from build123d import *

# Parameters (mm, degrees)
F0_W      = 500
F0_H      = 240
F0_W_2    = 420
F0_H_2    = 160
F1_DEPTH  = 40
F2_W      = 25
F2_H      = 360
F3_DEPTH  = 25
F4_W      = 400
F4_H      = 130
F4_W_2    = 350
F4_H_2    = 80
F5_DEPTH  = 25
F6_R      = 25
F6_R_2    = 22
F7_DEPTH  = 240
F11_R     = 20
F13_W     = 20
F13_H     = 100
F15_R     = 15
F16_DEPTH = 493.7865093372


with BuildPart() as f1:
    # F0 (on Top) → F1 (new body)
    with BuildSketch(Plane.XY):
        with Locations((250, 120)):
            Rectangle(F0_W, F0_H)
        with Locations((250, 120)):
            Rectangle(F0_W_2, F0_H_2, mode=Mode.SUBTRACT)
    extrude(amount=F1_DEPTH)

    # F2 (on face) → F3 (join)
    with BuildSketch(Plane.YZ.offset(500)):
        with Locations((67.5, 220)):
            Rectangle(F2_W, F2_H)
        with Locations((172.5, 220)):
            Rectangle(F2_W, F2_H)
    extrude(amount=-F3_DEPTH)

    # F4 (on face) → F5 (join)
    with BuildSketch(Plane.XY.offset(400)):
        with Locations((675, 120)):
            Rectangle(F4_W, F4_H)
        with Locations((675, 120)):
            Rectangle(F4_W_2, F4_H_2, mode=Mode.SUBTRACT)
    extrude(amount=F5_DEPTH)

    # F6 (on Front) → F7 (join)
    with BuildSketch(Plane.XZ):
        with Locations((524.9, 20)):
            Circle(F6_R)
        with Locations((524.9, 20)):
            Circle(F6_R_2, mode=Mode.SUBTRACT)
    extrude(amount=-F7_DEPTH)

    # F12: sweep along a path in F9
    with BuildLine(Plane.XZ.offset(-120)) as f12_path:
        Line((20, 20), (20, 102.3673019292))
        ThreePointArc((20, 102.3673019292), (18.4807753012, 119.7321196958), (13.9692620786, 136.5693162617))
        Line((13.9692620786, 136.5693162617), (-73.2424090723, 376.1814134616))
        ThreePointArc((-73.2424090723, 376.1814134616), (-96.5009930322, 412.6900772477), (-133.0096568183, 435.9486612076))
        Line((-133.0096568183, 435.9486612076), (-183.1603323585, 454.2020143326))
    # F11 (on line) → F12 (sweep)
    with BuildSketch(Plane.XY.offset(20)):
        with Locations((20, 120)):
            Circle(F11_R)
    sweep(path=f12_path.line)

    # F13 (on face) → F14 (revolve)
    with BuildSketch(Plane(origin=(-307.7123571346, 0, 111.9981387129), x_dir=(0, -1, 0), z_dir=(-0.9396926208, 0, 0.3420201433))):
        with Locations((-130, 364.1657580896)):
            Rectangle(F13_W, F13_H)
    revolve(axis=Axis((-183.1603323585, 120, 454.2020143326), (-0.3420201433, 0, -0.9396926208)))

    # F15 (on face) → F16 (cut, through all)
    with BuildSketch(Plane(origin=(141.6530319424, 0, 389.188506659), x_dir=(0.9396926208, 0, -0.3420201433), z_dir=(0.3420201433, 0, 0.9396926208))):
        with Locations((-327.4606507788, 120)):
            Circle(F15_R)
    extrude(amount=-F16_DEPTH, mode=Mode.SUBTRACT)


solid = f1.part
Can you work these out from the model? Positions are in its coordinate system, mm. A direction names the side the tool comes from. Give positions to 0.01 mm unless a question says otherwise; leave off trailing zeros. Loops run counter-clockwise (first coordinate to the right, second up) from the corner with the lowest first, then second, coordinate; pieces in that order, holes last. Notation, with made-up numbers: (-34.5, -18) - (-2.5, -18) arc R22 cw to (-2.5, 5) - close; hole circle Ø10 at (-27, 12). An arc over 180 degrees is marked (long way). Answer as a JSON object with one key per item and string values.
Q1. If we mould it in two halves opening along Y, with no side actions, what happens to faces 1 (the flat face through (585, 55, 403)), 2 (the flat face through (673, 160, 412)), 3 (the cylindrical face through (4, 108, 72)), 4 (the flat face through (685, 78, 400))? For each: pulls with the +Y half, pulls with the -Y half, needs draft (parallel to the pull), parting line crosses it, or undercut.
Geometry says:
{"face 1": "pulls with the -Y half", "face 2": "undercut", "face 3": "parting line crosses it", "face 4": "needs draft"}
Q2. Imagine slicing it at A-A on x = 425.5. Write out the boundary of the cut face in (y, z).
Geometry says:
{"outline": "(0, 0) - (40, 0) - (40, 40) - (0, 40) - close; (200, 0) - (240, 0) - (240, 40) - (200, 40) - close"}
Q3. Will these pins go through, and if not, where does the flat tip stop? P1, Ø3, axis at y = 170.5, z = 173, coming from the -X side; P2, Ø7.5, axis at x = 493.5, z = 205, coming from the +Y side; P3, Ø7.5, axis at y = 101.5, z = 413.5, coming from the -X side.
Geometry says:
{"P1": "x = 475", "P2": "y = 185", "P3": "x = -212.55"}
Q4. Which directions (+Z, -Z, +X, -X, +Y, -Y) give clear straight access to the entire face, cutting with the end or side of a thin tool? Please do faces 5 (the flat face through (460, 119, 20)), 6 (the cylindrical face through (-146.5, 112.3, 460.5)), 7 (the flat face through (487, 121, 400)).
Geometry says:
{"face 5": "+Z, -Z", "face 6": "none", "face 7": "+X"}
Q5. If I drill on L1, parallel to Y at x = 496.5, z = 228; L2, parallel to Z at x = 223, y = 209; L3, parallel to Z at x = 524.9, y = 153, over which ranges is the centre line in solid material (lowest first)?
Geometry says:
{"L1": "55 to 80, 160 to 185", "L2": "0 to 40", "L3": "-5 to -2, 42 to 45"}
Q6. Imagine slicing it at B-B on y = 219.5. Write out the boundary of the cut face in (x, z).
Geometry says:
{"outline": "(0, 0) - (500, 0) - (500, 17.77) arc R25 ccw (long way) to (500, 22.23) - (500, 40) - (0, 40) - close; hole circle Ø44 at (524.9, 20)"}
Q7. Imagine slicing it at C-C on z = 292. Give the number of separate pieces and of enclosed holes in the cut face, plus the area to 3 significant figures.
Geometry says:
{"separate pieces": "3", "enclosed holes": "0", "area": "2,590 mm²"}
